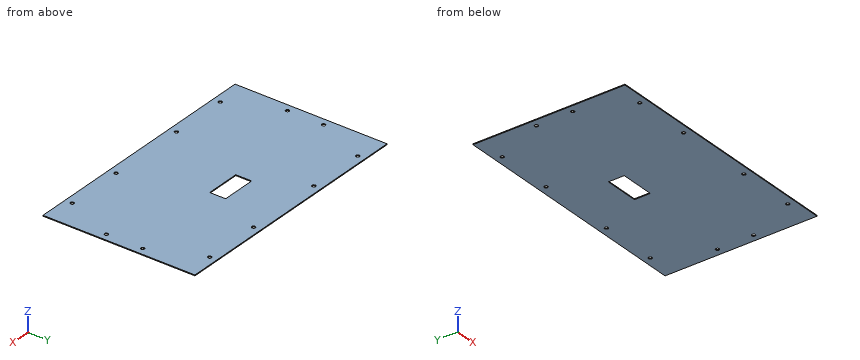
from build123d import *

# Parameters (mm, degrees)
SURFACE_EXTRUDE1_1_DEPTH = 350
THICKEN1_T1              = 1.2
SKETCH2_W                = 47.5
SKETCH2_H                = 22
CUT_EXTRUDE1_DEPTH       = 10
SKETCH3_R                = 2.5
CUT_EXTRUDE2_DEPTH       = 10


with BuildPart() as body_1:
    # Surface-Extrude1: a surface, the sketch's curves swept straight by 350 mm
    with BuildLine(Plane(origin=(0, 0, 0), x_dir=(0, 0, -1), z_dir=(1, 0, 0)), mode=Mode.PRIVATE) as surface_extrude1_1_path:
        Line((0, 0), (0, 210))
    surface_extrude1_1 = Shell.extrude(surface_extrude1_1_path.wire(), (1 * SURFACE_EXTRUDE1_1_DEPTH, 0 * SURFACE_EXTRUDE1_1_DEPTH, 0 * SURFACE_EXTRUDE1_1_DEPTH))
    add(Solid.thicken(surface_extrude1_1, THICKEN1_T1))

    # Sketch2 → Cut-Extrude1 (cut)
    with BuildSketch(Plane.XY.offset(1.2)):
        with Locations((176.75, 128)):
            Rectangle(SKETCH2_W, SKETCH2_H)
    extrude(amount=-CUT_EXTRUDE1_DEPTH, mode=Mode.SUBTRACT)

    # Sketch3 → Cut-Extrude2 (cut)
    with BuildSketch(Plane(origin=(0, 0, 0), x_dir=(-1, 0, 0), z_dir=(0, 0, -1))):
        with Locations((-310, 200)):
            Circle(SKETCH3_R)
        with Locations((-230, 200)):
            Circle(SKETCH3_R)
        with Locations((-340, 130)):
            Circle(SKETCH3_R)
        with Locations((-10, 130)):
            Circle(SKETCH3_R)
        with Locations((-120, 200)):
            Circle(SKETCH3_R)
        with Locations((-40, 200)):
            Circle(SKETCH3_R)
        with Locations((-10, 80)):
            Circle(SKETCH3_R)
        with Locations((-40, 10)):
            Circle(SKETCH3_R)
        with Locations((-120, 10)):
            Circle(SKETCH3_R)
        with Locations((-230, 10)):
            Circle(SKETCH3_R)
        with Locations((-310, 10)):
            Circle(SKETCH3_R)
        with Locations((-340, 80)):
            Circle(SKETCH3_R)
    extrude(amount=-CUT_EXTRUDE2_DEPTH, mode=Mode.SUBTRACT)


solid = body_1.part
Check sheet for the modelled part. Datum: model origin and axes. Units: mm. Round coordinates to 2 decimals unless told otherwise and drop trailing zeros. Loops run counter-clockwise (first coordinate to the right, second up) from the corner with the lowest first, then second, coordinate; pieces in that order, holes last.
1. Sectioned sample at A-A on x = 177.5. Record the boundary of the cut face in (y, z), and give its area (3 significant figures).
2. Sectioned sample at B-B on z = 0.7. Give the number of separate pieces and of enclosed holes in the cut face, and give its area (3 significant figures).
3. Scan lines: probe 1 along X at (y, z) = (130, 0.8); probe 2 along Y at (x, z) = (10, 0.3); probe 3 along X at (y, z) = (200, 0.65). Record each from-to range of solid material in increasing order.
4. Gauge pin test, flat ends, axial feed: pin 1 Ø5 at (x, y) = (183, 98) entering from -Z; pin 2 Ø4 at (x, y) = (40, 10) entering from +Z. Record the tip position at first contact, or that the pin passes through.
Recorded:
1. outline: (0, 0) - (117, 0) - (117, 1.2) - (0, 1.2) - close; (139, 0) - (210, 0) - (210, 1.2) - (139, 1.2) - close
1. area: 226 mm2
2. separate pieces: 1
2. enclosed holes: 13
2. area: 72,200 mm2
3. probe 1: x = 0 to 7.5, 12.5 to 153, 200.5 to 337.5, 342.5 to 350
3. probe 2: y = 0 to 77.5, 82.5 to 127.5, 132.5 to 210
3. probe 3: x = 0 to 37.5, 42.5 to 117.5, 122.5 to 227.5, 232.5 to 307.5, 312.5 to 350
4. pin 1: stops at z = 0
4. pin 2: passes through
